from build123d import *

# Parameters (mm, degrees)
EXTRUDE_1_DEPTH     = 9
EXTRUDE_2_DEPTH     = 13
SKETCH_5_R          = 4.25
CUT_EXTRUDE_1_DEPTH = 7


with BuildPart() as part:
    # Эскиз1 → Повернуть1 (revolve)
    with BuildSketch(Plane.XY, mode=Mode.PRIVATE) as revolve_1_sk:
        Polygon((0, 0), (-30, 0), (-30, 6), (-17, 6), (-16, 20), (-12, 20), (-12, 22), (-8, 26), (-8, 29), (-8, 38), (-8, 136), (-6, 138), (0, 138), align=None)
    revolve(revolve_1_sk.sketch.rotate(Axis((0, 0, 0), (0, 1, 0)), 180), axis=Axis((0, 0, 0), (0, 1, 0)))  # turned: the seam where the file's is

    # Эскиз2 → Бобышка-Вытянуть1 (add)
    with BuildSketch(Plane(origin=(0, 29, 0), x_dir=(1, 0, 0), z_dir=(0, 1, 0))):
        Polygon((0, 13.856406461), (-12, 6.92820323), (-12, -6.92820323), (0, -13.856406461), (12, -6.92820323), (12, 6.92820323), align=None)
    extrude(amount=EXTRUDE_1_DEPTH)

    # Эскиз3 → Бобышка-Вытянуть2 (add)
    with BuildSketch(Plane(origin=(0, 87, 0), x_dir=(1, 0, 0), z_dir=(0, 1, 0))):
        Polygon((12, 6.92820323), (0, 13.856406461), (-12, 6.92820323), (-12, -6.92820323), (0, -13.856406461), (12, -6.92820323), align=None)
    extrude(amount=EXTRUDE_2_DEPTH)

    # Эскиз4 → Вырез-Повернуть2 (revolve, cut)
    with BuildSketch(Plane.XY, mode=Mode.PRIVATE) as cut_revolve_2_sk:
        Polygon((-23.258330249, 100), (-12, 100), (-23.258330249, 93.5), align=None)
        Polygon((-23.258330249, 87), (-23.258330249, 93.5), (-12, 87), align=None)
        Polygon((-19.794228634, 38), (-19.794228634, 33.5), (-12, 38), align=None)
        Polygon((-19.794228634, 33.5), (-19.794228634, 29), (-12, 29), align=None)
    revolve(cut_revolve_2_sk.sketch.rotate(Axis((0, 138, 0), (0, -1, 0)), 180), axis=Axis((0, 138, 0), (0, -1, 0)), mode=Mode.SUBTRACT)  # turned: the seam where the file's is

    # Эскиз5 → Вырез-Вытянуть1 (cut, through all)
    with BuildSketch(Plane(origin=(0, 6, 0), x_dir=(1, 0, 0), z_dir=(0, 1, 0))):
        with Locations(Location((-23.75, 0, 0), (0, 0, 180))):  # turned: the seam where the file's is
            Circle(SKETCH_5_R)
        with Locations(Location((23.75, 0, 0), (0, 0, 180))):  # turned: the seam where the file's is
            Circle(SKETCH_5_R)
    extrude(amount=-CUT_EXTRUDE_1_DEPTH, mode=Mode.SUBTRACT)


solid = part.part
Work out the finished part from the listing and answer in its coordinate system (mm). A direction names the side the tool comes from. Give positions to 0.01 mm unless a question says otherwise; leave off trailing zeros. Order: outer loops, then holes, each group sorted by start corner. A loop starts at its lowest first (then second) coordinate and runs counter-clockwise, first axis right, second up. Notation, with made-up numbers: (6.25, 5) -> (55.25, 5) arc R26 ccw to (55.25, 20) -> close; hole circle Ø1 at (-8, 11). An arc over 180 degrees is marked (long way). Answer as a JSON object with one key per item and string values. Group by question number.
1. Consider line 1 along Y through (x, z) = (0, 13.5); line 2 along Y through (x, z) = (-11.5, -5); line 3 along Y through (x, z) = (-4, -25.5). Determine where each line is inside the solid, lowest interval first. Write a range as [from, to].
2. Section D-D on x = 10 is taken. Count the separate pieces of the cut face and the enclosed holes in it, plus the area to 3 significant figures.
3. The mould has two halves that part along Y. Classify faces 5 (the conical face through (-10.791, 37.744, -6.195)), 6 (the conical face through (-0.03, 99.74, -12.45)), 7 (the cylindrical face through (-1.73, 27.48, 7.81)), 8 (the flat face through (6.084, 33.437, -10.344)): released by +Y, released by -Y, zero draft, split by the parting line, or undercut.
4. Section C-C on z = -23 is taken. Determine the outline of the cut face in (x, y).
5. Section A-A on x = -23.75 is taken. Determine the outline of the cut face in (y, z).
6. A tool of negligible diameter and unlimited length cuts with its end or side. For faces 1 (the conical face through (-0.03, 37.744, -12.443)), 2 (the flat face through (2, 38, 8)), 3 (the flat face through (6.084, 93.409, -10.344)), 4 (the conical face through (10.77, 29.26, -6.25)), from which of +Z, -Z, +X, -X, +Y, -Y can it reach the whole face along a straight path? Write none if from no direction.
7. Section B-B on y = 128 is taken. Determine the outline of the cut face in (x, z).
8. Flat-ended cylindrical pins translate along their axes: pin 1 Ø2.5 at (y, z) = (35.5, 2.5) entering from +X; pin 2 Ø2 at (y, z) = (46.5, -10.5) entering from +X; pin 3 Ø1 at (x, y) = (3.5, 107) entering from +Z; pin 4 Ø7 at (y, z) = (34.5, -2) entering from -X. Find the tip coordinate at first contact, or state that the pin passes through.
Result sheet:
{
 "1": {"line 1": "y = [0, 20], [29.87, 37.13], [87.87, 99.13]", "line 2": "y = [0, 20], [29.31, 37.69], [87.31, 99.69]", "line 3": "y = [0, 6]"},
 "2": {"separate pieces": "3", "enclosed holes": "0", "area": "1,100 mm^2"},
 "3": {"face 5": "undercut", "face 6": "released by +Y", "face 7": "undercut", "face 8": "zero draft"},
 "4": {"outline": "(-19.26, 0) -> (19.26, 0) -> (19.26, 6) -> (-19.26, 6) -> close"},
 "5": {"outline": "(0, -18.33) -> (6, -18.33) -> (6, -4.25) -> (0, -4.25) -> close; (0, 4.25) -> (6, 4.25) -> (6, 18.33) -> (0, 18.33) -> close"},
 "6": {"face 1": "-Z", "face 2": "none", "face 3": "-Z, +X, +Y", "face 4": "-Z, +X"},
 "7": {"outline": "circle Ø16 at (0, 0)"},
 "8": {"pin 1": "stops at x = 12", "pin 2": "passes through", "pin 3": "stops at z = 7.42", "pin 4": "stops at x = -12"}
}
